```python
from build123d import *

# Parameters (mm, degrees)
SKETCH1_R           = 8
BOSS_EXTRUDE1_DEPTH = 13
SKETCH2_R           = 8.75
BOSS_EXTRUDE2_DEPTH = 2
SKETCH3_W           = 49
SKETCH3_H           = 62.5
BOSS_EXTRUDE3_DEPTH = 15
SKETCH4_R           = 17.65
BOSS_EXTRUDE4_DEPTH = 27.3
BOSS_EXTRUDE6_DEPTH = 36.5
SKETCH7_W           = 81.110714311
SKETCH7_H           = 82.460514398
CUT_EXTRUDE1_DEPTH  = 31
CUT_EXTRUDE2_DEPTH  = 14
SKETCH9_R           = 2.5
CUT_EXTRUDE4_DEPTH  = 17
SKETCH10_R          = 1.6
CUT_EXTRUDE5_DEPTH  = 17
FILLET1_R           = 0.5
SKETCH11_W          = 6
SKETCH11_H          = 2.1
CUT_EXTRUDE6_DEPTH  = 12


with BuildPart() as part:
    # Sketch1 → Boss-Extrude1 (new body)
    with BuildSketch(Plane.XY):
        Circle(SKETCH1_R)
    extrude(amount=BOSS_EXTRUDE1_DEPTH)

    # Sketch2 → Boss-Extrude2 (add)
    with BuildSketch(Plane.XY.offset(13)):
        Circle(SKETCH2_R)
    extrude(amount=BOSS_EXTRUDE2_DEPTH)

    # Sketch3 → Boss-Extrude3 (add)
    with BuildSketch(Plane.XY.offset(15)):
        with Locations((0, -13.38)):
            Rectangle(SKETCH3_W, SKETCH3_H)
    extrude(amount=BOSS_EXTRUDE3_DEPTH)

    # Sketch4 → Boss-Extrude4 (add)
    with BuildSketch(Plane(origin=(0, 0, 15), x_dir=(-1, 0, 0), z_dir=(0, 0, -1))):
        with Locations((0, -29.5)):
            Circle(SKETCH4_R)
    extrude(amount=-BOSS_EXTRUDE4_DEPTH)

    # Sketch6 → Boss-Extrude6 (add)
    with BuildSketch(Plane(origin=(0, 0, 0), x_dir=(-1, 0, 0), z_dir=(0, 0, -1))):
        with BuildLine():
            Line((2, 1.5), (-2, 1.5))
            ThreePointArc((-2, 1.5), (-2.5, 0), (-2, -1.5))
            Line((-2, -1.5), (2, -1.5))
            ThreePointArc((2, -1.5), (2.371708245, -0.790569415), (2.5, 0))
            ThreePointArc((2.5, 0), (2.371708245, 0.790569415), (2, 1.5))
        make_face()
    extrude(amount=-BOSS_EXTRUDE6_DEPTH)

    # Sketch7 → Cut-Extrude1 (cut, through all)
    with BuildSketch(Plane.XY.offset(30)):
        with Locations((0.873030834, -13.704939381)):
            Rectangle(SKETCH7_W, SKETCH7_H)
        with BuildLine():
            Line((-8, 17.87), (8, 17.87))
            Line((8, 17.87), (8, 12.87))
            Line((8, 12.87), (8.5, 12.87))
            ThreePointArc((8.5, 12.87), (13.803300859, 10.673300859), (16, 5.37))
            Line((16, 5.37), (16, 2.87))
            Line((16, 2.87), (19.5, -10))
            Line((19.5, -10), (22.5, -10))
            ThreePointArc((22.5, -10), (23.914213562, -10.585786438), (24.5, -12))
            Line((24.5, -12), (24.5, -31))
            ThreePointArc((24.5, -31), (23.914213562, -32.414213562), (22.5, -33))
            Line((22.5, -33), (17.299494212, -33))
            ThreePointArc((17.299494212, -33), (0, -47.15), (-17.299494212, -33))
            Line((-17.299494212, -33), (-22.5, -33))
            ThreePointArc((-22.5, -33), (-23.914213562, -32.414213562), (-24.5, -31))
            Line((-24.5, -31), (-24.5, -12))
            ThreePointArc((-24.5, -12), (-23.914213562, -10.585786438), (-22.5, -10))
            Line((-22.5, -10), (-19.5, -10))
            Line((-19.5, -10), (-16, 2.87))
            Line((-16, 2.87), (-16, 5.37))
            ThreePointArc((-16, 5.37), (-13.803300859, 10.673300859), (-8.5, 12.87))
            Line((-8.5, 12.87), (-8, 12.87))
            Line((-8, 12.87), (-8, 17.87))
        make_face(mode=Mode.SUBTRACT)
    extrude(amount=-CUT_EXTRUDE1_DEPTH, mode=Mode.SUBTRACT)

    # Sketch8 → Cut-Extrude2 (cut)
    with BuildSketch(Plane.XY.offset(30)):
        with BuildLine():
            Line((-17.299494212, -33), (-22.5, -33))
            ThreePointArc((-22.5, -33), (-23.914213562, -32.414213562), (-24.5, -31))
            Line((-24.5, -31), (-24.5, -12))
            ThreePointArc((-24.5, -12), (-23.914213562, -10.585786438), (-22.5, -10))
            Line((-22.5, -10), (22.5, -10))
            ThreePointArc((22.5, -10), (23.914213562, -10.585786438), (24.5, -12))
            Line((24.5, -12), (24.5, -31))
            ThreePointArc((24.5, -31), (23.914213562, -32.414213562), (22.5, -33))
            Line((22.5, -33), (17.299494212, -33))
            ThreePointArc((17.299494212, -33), (0, -11.85), (-17.299494212, -33))
        make_face()
    extrude(amount=-CUT_EXTRUDE2_DEPTH, mode=Mode.SUBTRACT)

    # Sketch9 → Cut-Extrude4 (cut, through all)
    with BuildSketch(Plane.XY.offset(16)):
        with Locations((-21, -21.5)):
            Circle(SKETCH9_R)
        with Locations((21, -21.5)):
            Circle(SKETCH9_R)
    extrude(amount=-CUT_EXTRUDE4_DEPTH, mode=Mode.SUBTRACT)

    # Sketch10 → Cut-Extrude5 (cut, through all)
    with BuildSketch(Plane.XY.offset(16)):
        with Locations((-21, -13.5)):
            Circle(SKETCH10_R)
        with Locations((21, -13.5)):
            Circle(SKETCH10_R)
        with Locations((21, -29.5)):
            Circle(SKETCH10_R)
        with Locations((-21, -29.5)):
            Circle(SKETCH10_R)
    extrude(amount=-CUT_EXTRUDE5_DEPTH, mode=Mode.SUBTRACT)

    # Fillet1
    fillet1_edges = [part.edges().sort_by_distance(p)[0] for p in [
        (-8, 0, 0),
    ]]
    fillet(fillet1_edges, radius=FILLET1_R)

    # Sketch11 → Cut-Extrude6 (cut)
    with BuildSketch(Plane(origin=(0, 0, 0), x_dir=(-1, 0, 0), z_dir=(0, 0, -1))):
        Rectangle(SKETCH11_W, SKETCH11_H)
    extrude(amount=-CUT_EXTRUDE6_DEPTH, mode=Mode.SUBTRACT)


solid = part.part
```
For this review, take the finished solid that the model builds, in its own axes (mm). A direction names the side the tool comes from. Give positions to 0.01 mm unless a question says otherwise; leave off trailing zeros. Order: outer loops, then holes, each group sorted by start corner. A loop starts at its lowest first (then second) coordinate and runs counter-clockwise, first axis right, second up.
1) Take a section at A-A (y = -29.5). Give the boundary of the cut face in (x, z), then the cut area to 3 significant figures.
2) Take a section at B-B (z = 18.5). Give the boundary of the cut face in (x, y), then the cut area to 3 significant figures.
3) Take a section at D-D (x = 0). Give the boundary of the cut face in (y, z), then the cut area to 3 significant figures.
4) Take a section at C-C (x = 21). Give the boundary of the cut face in (y, z).
5) Wall thickness on line 1 (Y direction, x = 21, z = 15.5); line 2 (Y direction, x = 0.5, z = 33); line 3 (Z direction, x = 5, y = -1): over which ranges is each line inside the solid? List them lowest first.
6) For faces 1 (the face through (-1.73, -7.81, 6.66)), 2 (the face through (0, 17.87, 22)), 3 (the face through (0, 0, 36.5)), 4 (the face through (4, -12, 16)), 5 (the face through (-8, 15, 23)), list the 3-axis set-ups (+Z, -Z, +X, -X, +Y, -Y) from which the entire face can be reached by the end or side of a thin tool; tool diameter is ignored.
7) Insertion check: pin 1 (1 mm diameter, centred on x = 5, y = 9.5, fed in from +Z); pin 2 (8 mm diameter, centred on x = -21, y = -21.5, fed in from +Z); pin 3 (2 mm diameter, centred on x = 18, y = -21, fed in from -Z); pin 4 (8 mm diameter, centred on y = -21.5, z = 10.5, fed in from -X). Each pin has a flat end and moves straight along its axis. Give the tip position at first contact, or say it passes through.
8) The part is to be moulded in two halves that separate along Y. For faces 6 (the face through (16, 4, 23)), 7 (the face through (-23.93, -10.6, 15.51)), 8 (the face through (20.792, -27.914, 15.507)), say which applies: released by +Y, released by -Y, zero draft, split by the parting line, or undercut.
Derived:
1. outline: (-24.5, 15) - (-22.6, 15) - (-22.6, 16) - (-24.5, 16) - close; (-19.4, 15) - (19.4, 15) - (19.4, 16) - (17.65, 16) - (17.65, 42.3) - (-17.65, 42.3) - (-17.65, 16) - (-19.4, 16) - close; (22.6, 15) - (24.5, 15) - (24.5, 16) - (22.6, 16) - close
1. area: 971 mm2
2. outline: (-19.5, -10) - (19.5, -10) - (16, 2.87) - (16, 5.37) arc R7.5 ccw to (8.5, 12.87) - (8, 12.87) - (8, 17.87) - (-8, 17.87) - (-8, 12.87) - (-8.5, 12.87) arc R7.5 ccw to (-16, 5.37) - (-16, 2.87) - close; circle Ø35.3 at (0, -29.5)
2. area: 1,810 mm2
3. outline: (-47.15, 15) - (-8.75, 15) - (-8.75, 13) - (-8, 13) - (-8, 0.5) arc R0.5 ccw to (-7.5, 0) - (-1.05, 0) - (-1.05, 12) - (1.05, 12) - (1.05, 0) - (7.5, 0) arc R0.5 ccw to (8, 0.5) - (8, 13) - (8.75, 13) - (8.75, 15) - (17.87, 15) - (17.87, 30) - (1.5, 30) - (1.5, 36.5) - (-1.5, 36.5) - (-1.5, 30) - (-10, 30) - (-10, 16) - (-11.85, 16) - (-11.85, 42.3) - (-47.15, 42.3) - close
3. area: 1,620 mm2
4. outline: (-33, 15) - (-31.1, 15) - (-31.1, 16) - (-33, 16) - close; (-27.9, 15) - (-24, 15) - (-24, 16) - (-27.9, 16) - close; (-19, 15) - (-15.1, 15) - (-15.1, 16) - (-19, 16) - close; (-11.9, 15) - (-10, 15) - (-10, 16) - (-11.9, 16) - close
5. line 1: y = -33 to -31.1, -27.9 to -24, -19 to -15.1, -11.9 to -10
5. line 2: y = -47.14 to -11.86, -1.5 to 1.5
5. line 3: z = 0 to 30
6. face 1: -Z
6. face 2: +Z, -Z, +X, -X, +Y
6. face 3: +Z, +X, -X, +Y
6. face 4: +Z
6. face 5: +Z, -Z, -X, +Y
7. pin 1: stops at z = 30
7. pin 2: stops at z = 16
7. pin 3: stops at z = 15
7. pin 4: passes through
8. face 6: zero draft
8. face 7: released by +Y
8. face 8: undercut
